Source: CAD feature listing. Evaluate the final solid. Frame: model axes, mm. Face numbers are marked on the shaded views. A direction names the side the tool comes from. Give positions to 0.01 mm unless a question says otherwise; leave off trailing zeros. Order: outer loops, then holes, each group sorted by start corner. A loop starts at its lowest first (then second) coordinate and runs counter-clockwise, first axis right, second up. Notation, with made-up numbers: M 46.5,2.25 L 79.5,2.25 A12 cw 79.5,13.25 Z; hole C -22.5,1 d6. An arc over 180 degrees is marked long. Answer as a JSON object with one key per item and string values. Group by question number.
1. Section query A-A (x = 0). Output: boundary loops of the cut face in (y, z), plus the area to 3 significant figures.
2. Section query B-B (z = -12.5). Output: boundary loops of the cut face in (x, y), plus the area to 3 significant figures.
3. Set-up query: the marked faces 1 and 2. Return all of +Z, -Z, +X, -X, +Y, -Y with unobstructed straight access to the full face (end or side cutting, diameter ignored); none if empty.
4. Pin query (flat end, axial travel): P1, Ø3, axis at x = -8, z = -4.5, coming from the -Y side. Return the tip coordinate at first contact, or that it passes through.
5. Section query D-D (z = -20.5). Output: boundary loops of the cut face in (x, y), plus the area to 3 significant figures.
6. Material intervals for L1, parallel to Z at x = -18, y = -1; L2, parallel to X at y = 3.15, z = -4.5; L3, parallel to Z at x = 8, y = 3.3, sorted ascending. Write a range as [from, to].
7. Section query C-C (y = -1). Output: boundary loops of the cut face in (x, z), plus the area to 3 significant figures.
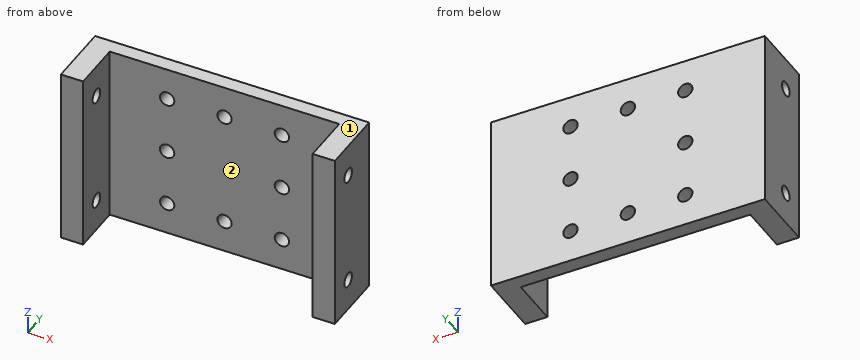
Solid Edge part; units mm, degrees
sketch "Sketch1" plane through (0, 0, 0) normal (0, 0, -1) x (-1, 0, 0)
  line L0 (19.1, -4.5) -> (-19.1, -4.5)
  line L1 (-19.1, -4.5) -> (-19.1, 4.5)
  line L2 (-19.1, 4.5) -> (19.1, 4.5)
  line L3 (19.1, 4.5) -> (19.1, -4.5)
  dimension "D1" = 19.1
  dimension "D2" = 19.1
extrude "Protrusion1" add sketch "Sketch1" along normal blind 25
sketch "Sketch2" plane through (0, 0, -25) normal (0, 0, -1) x (1, 0, 0)
  line L0 (-16, 4.5) -> (16, 4.5)
  line L1 (16, 4.5) -> (16, -2.5)
  line L2 (16, -2.5) -> (-16, -2.5)
  line L3 (-16, -2.5) -> (-16, 4.5)
  dimension "D1" = 16
  dimension "D2" = 16
extrude "Cutout1" cut sketch "Sketch2" against normal through all
hole "Hole_1" at (-19.1, -1, -4.5) direction (1, 0, 0) diameter 2 end through all
hole "Hole1" at (-19.1, -1, -20.5) direction (1, 0, 0) diameter 2 end through all
hole "Hole_3" at (0, 4.5, -20.5) direction (0, -1, 0) diameter 2 end through all
hole "Hole2" at (0, 4.5, -4.5) direction (0, -1, 0) diameter 2 end through all
hole "Hole3" at (-8, 4.5, -4.5) direction (0, -1, 0) diameter 2 end through all
hole "Hole4" at (-8, 4.5, -12.5) direction (0, -1, 0) diameter 2 end through all
hole "Hole5" at (-8, 4.5, -20.5) direction (0, -1, 0) diameter 2 end through all
hole "Hole6" at (8, 4.5, -20.5) direction (0, -1, 0) diameter 2 end through all
hole "Hole7" at (8, 4.5, -12.5) direction (0, -1, 0) diameter 2 end through all
hole "Hole8" at (8, 4.5, -4.5) direction (0, -1, 0) diameter 2 end through all
Answer sheet:
{
 "1": {"outline": "M 2.5,-25 L 4.5,-25 L 4.5,-21.5 L 2.5,-21.5 Z; M 2.5,-19.5 L 4.5,-19.5 L 4.5,-5.5 L 2.5,-5.5 Z; M 2.5,-3.5 L 4.5,-3.5 L 4.5,0 L 2.5,0 Z", "area": "42.0 mm^2"},
 "2": {"outline": "M -19.1,-4.5 L -16,-4.5 L -16,2.5 L -9,2.5 L -9,4.5 L -19.1,4.5 Z; M -7,2.5 L 7,2.5 L 7,4.5 L -7,4.5 Z; M 9,2.5 L 16,2.5 L 16,-4.5 L 19.1,-4.5 L 19.1,4.5 L 9,4.5 Z", "area": "112 mm^2"},
 "3": {"face 1": "+Z, +X, -X, +Y, -Y", "face 2": "+Z, -Z, -Y"},
 "4": {"P1": "y = 2.5"},
 "5": {"outline": "M -19.1,-4.5 L -16,-4.5 L -16,-2 L -19.1,-2 Z; M -19.1,0 L -16,0 L -16,2.5 L -9,2.5 L -9,4.5 L -19.1,4.5 Z; M -7,2.5 L -1,2.5 L -1,4.5 L -7,4.5 Z; M 1,2.5 L 7,2.5 L 7,4.5 L 1,4.5 Z; M 9,2.5 L 16,2.5 L 16,0 L 19.1,0 L 19.1,4.5 L 9,4.5 Z; M 16,-4.5 L 19.1,-4.5 L 19.1,-2 L 16,-2 Z", "area": "95.4 mm^2"},
 "6": {"L1": "[-25, -21.5], [-19.5, -5.5], [-3.5, 0]", "L2": "[-19.1, -9], [-7, -1], [1, 7], [9, 19.1]", "L3": "[-25, -21.5], [-19.5, -13.5], [-11.5, -5.5], [-3.5, 0]"},
 "7": {"outline": "M -19.1,-25 L -16,-25 L -16,-21.5 L -19.1,-21.5 Z; M -19.1,-19.5 L -16,-19.5 L -16,-5.5 L -19.1,-5.5 Z; M -19.1,-3.5 L -16,-3.5 L -16,0 L -19.1,0 Z; M 16,-25 L 19.1,-25 L 19.1,-21.5 L 16,-21.5 Z; M 16,-19.5 L 19.1,-19.5 L 19.1,-5.5 L 16,-5.5 Z; M 16,-3.5 L 19.1,-3.5 L 19.1,0 L 16,0 Z", "area": "130 mm^2"}
}
